The model under review builds one solid part; all positions refer to its coordinate system, in mm. A direction names the side the tool comes from. Round coordinates to 2 decimals unless told otherwise and drop trailing zeros. Write each loop counter-clockwise with the first axis right and the second up, starting at its lowest first coordinate (ties: lowest second). Pieces come first, ordered by that corner, then holes.
Item 1: Add section A-A (y = 1.5). Give the boundary of the cut face in (x, z).
Item 2: To check wall thickness, follow L1, parallel to X at y = 1.4, z = 0; L2, parallel to Y at x = 41.5, z = 4; L3, parallel to X at y = -3.5, z = -0.25. State the ranges of each line that lie inside material, in increasing order.
Item 3: Machinability: for faces 4 (the face through (22, -10.5, 0)), 5 (the face through (5, -1.1, 0)), which of the approach directions +Z, -Z, +X, -X, +Y, -Y give a long, thin tool a straight path to every point of the face, cutting with its end or side? Answer none if there is none.
Item 4: Clearance check with flat-ended pins moving along their axes: pin 1 Ø6 at (x, y) = (31, -9) entering from +Z; pin 2 Ø1.5 at (x, z) = (2.5, -2) entering from -Y; pin 3 Ø0.9 at (y, z) = (-0.5, -2.5) entering from +X; pin 4 Ø3 at (y, z) = (-9, -3) entering from +X. State where each tip first meets the part, or that it passes through.
Item 5: Add section B-B (z = 0). State how many separate pieces and enclosed holes the cut face has, plus the area to 3 significant figures.
Item 6: Draft analysis for pull direction X (two halves, no side actions). For faces 1 (the face through (44, 0, 0)), 2 (the face through (-55, 1, 0)), 3 (the face through (0.7, -0.8, 6)), state which applies: +X half, -X half, draft (parallel to the pull), parting line (faces both ways), or undercut.
Item 7: Add section C-C (x = 51.5). Give the boundary of the cut face in (y, z), plus the area to 3 significant figures.
Item 8: Add section D-D (y = -3.75). Give the boundary of the cut face in (x, z).
```python
from build123d import *

# Parameters (mm, degrees)
SKETCH1_R                 = 1.5
BOSS_EXTRUDE1_DEPTH       = 3
SKETCH4_W                 = 3.5
SKETCH4_H                 = 12
BOSS_EXTRUDE3_DEPTH       = 10.5
SKETCH5_W                 = 2
SKETCH5_H                 = 12
BOSS_EXTRUDE4_DEPTH       = 1.1
SKETCH6_W                 = 0.2
SKETCH6_H                 = 3
BOSS_EXTRUDE5_DEPTH       = 0.5
CHAMFER1_SIZE             = 10.5
F_3_0MM_DOWEL_HOLE1_D     = 3
F_3_0MM_DOWEL_HOLE1_DEPTH = 13.5


with BuildPart() as part:
    # Sketch1 → Boss-Extrude1 (new body)
    with BuildSketch(Plane(origin=(0, 0, 0), x_dir=(1, 0, 0), z_dir=(0, 1, 0))):
        with BuildLine():
            Line((-49, 6), (49, 6))
            ThreePointArc((49, 6), (55, 0), (49, -6))
            Line((49, -6), (-49, -6))
            ThreePointArc((-49, -6), (-55, 0), (-49, 6))
        make_face()
        with Locations(Location((-51.5, 0, 0), (0, 0, 270))):
            Circle(SKETCH1_R, mode=Mode.SUBTRACT)
        with Locations(Location((51.5, 0, 0), (0, 0, 270))):
            Circle(SKETCH1_R, mode=Mode.SUBTRACT)
    extrude(amount=BOSS_EXTRUDE1_DEPTH)

    # Sketch4 → Boss-Extrude3 (add)
    with BuildSketch(Plane.XZ):
        with Locations((-21.690023983, 0)):
            Rectangle(SKETCH4_W, SKETCH4_H)
        with Locations((21.690023983, 0)):
            Rectangle(SKETCH4_W, SKETCH4_H)
    extrude(amount=BOSS_EXTRUDE3_DEPTH)

    # Sketch5 → Boss-Extrude4 (add)
    with BuildSketch(Plane.XZ):
        with Locations((5, 0)):
            Rectangle(SKETCH5_W, SKETCH5_H)
        Rectangle(SKETCH5_W, SKETCH5_H)
        with Locations((10, 0)):
            Rectangle(SKETCH5_W, SKETCH5_H)
        with Locations((-5, 0)):
            Rectangle(SKETCH5_W, SKETCH5_H)
        with Locations((-10, 0)):
            Rectangle(SKETCH5_W, SKETCH5_H)
    extrude(amount=BOSS_EXTRUDE4_DEPTH)

    # Sketch6 → Boss-Extrude5 (add)
    with BuildSketch(Plane.XY.offset(6)):
        with Locations((48.9, 1.5)):
            Rectangle(SKETCH6_W, SKETCH6_H)
        with Locations((-48.9, 1.5)):
            Rectangle(SKETCH6_W, SKETCH6_H)
    extrude(amount=BOSS_EXTRUDE5_DEPTH)

    # Chamfer1
    chamfer1_edges = [part.edges().sort_by_distance(p)[0] for p in [
        (23.440023983, 0, 0),
        (-23.440023983, 0, 0),
    ]]
    chamfer(chamfer1_edges, length=CHAMFER1_SIZE - 0.0001)  # a hair under: the kernel refuses the full size

    # Ø3.0mm Dowel Hole1
    with Locations(Plane(origin=(0, 3, 0), x_dir=(1, 0, 0), z_dir=(0, 1, 0))):
        with Locations((-51.5, 0), (51.5, 0)):
            Hole(F_3_0MM_DOWEL_HOLE1_D / 2, depth=F_3_0MM_DOWEL_HOLE1_DEPTH)


solid = part.part
```
Numbers:
1. outline: (-49, -6) - (49, -6) arc R6 ccw to (49, 6) - (49, 6.5) - (48.8, 6.5) - (48.8, 6) - (-48.8, 6) - (-48.8, 6.5) - (-49, 6.5) - (-49, 6) arc R6 ccw to start; hole circle Ø3 at (-51.5, 0); hole circle Ø3 at (51.5, 0)
2. L1: x = -55 to -53, -50 to 50, 53 to 55
2. L2: y = 0 to 3
2. L3: x = -30.44 to -19.94, 19.94 to 30.44
3. face 4: +Z, -Z, +X, -X, -Y
3. face 5: +Z, -Z, -Y
4. pin 1: passes through
4. pin 2: stops at y = 0
4. pin 3: stops at x = 33.89
4. pin 4: stops at x = 26.44
5. separate pieces: 3
5. enclosed holes: 0
5. area: 507 mm2
6. face 1: draft
6. face 2: -X half
6. face 3: undercut
7. outline: (0, -5.45) - (3, -5.45) - (3, -1.5) - (0, -1.5) - close; (0, 1.5) - (3, 1.5) - (3, 5.45) - (0, 5.45) - close
7. area: 23.7 mm2
8. outline: (-30.19, -6) - (-19.94, -6) - (-19.94, 6) - (-30.19, 6) - close; (19.94, -6) - (30.19, -6) - (30.19, 6) - (19.94, 6) - close
